The model under review builds one solid part; all positions refer to its coordinate system, in mm. Round coordinates to 2 decimals unless told otherwise and drop trailing zeros. Order: outer loops, then holes, each group sorted by start corner. A loop starts at its lowest first (then second) coordinate and runs counter-clockwise, first axis right, second up. Notation, with made-up numbers: M 28,-33.75 L 52,-33.75 A26 ccw 52,-17.75 Z; hole C -40,-24.5 d4. An arc over 180 degrees is marked long. Answer as a JSON object with one key per item and string values. Group by question number.
1) Insertion check: pin 1 Ø1.5 at (y, z) = (11, 0.5) entering from +X; pin 2 Ø5 at (x, y) = (7.5, 9.5) entering from +Z. Each pin has a flat end and moves straight along its axis. Give the tip position at first contact, or say it passes through.
2) Consider section A-A, the plane z = 2.1. Write out the cut boundary in (x, y).
3) To check wall thickness, follow line 1 (X direction, y = 2.5, z = 1.8); line 2 (Y direction, x = 5, z = 3.75); line 3 (X direction, y = 7, z = 3.1). State the ranges of each line that lie inside material, in increasing order.
4) Consider section C-C, the plane x = 6. Write out the cut boundary in (y, z).
5) Consider section B-B, the plane y = 2. Write out the cut boundary in (x, z), then the cut area to 3 significant figures.
```python
from build123d import *

# Parameters (mm, degrees)
BOSS_EXTRUDE1_DEPTH = 4.7625


with BuildPart() as part:
    # Sketch1 → Boss-Extrude1 (new body)
    with BuildSketch(Plane.XY):
        with BuildLine():
            Line((0, 0), (12.758578644, 0))
            ThreePointArc((12.758578644, 0), (12.850966597, 0.061731657), (12.829289322, 0.170710678))
            Line((12.829289322, 0.170710678), (0.170710678, 12.829289322))
            ThreePointArc((0.170710678, 12.829289322), (0.061731657, 12.850966597), (0, 12.758578644))
            Line((0, 12.758578644), (0, 0))
        make_face()
    extrude(amount=BOSS_EXTRUDE1_DEPTH)


solid = part.part
```
Results list:
{
 "1": {"pin 1": "x = 2.75", "pin 2": "through"},
 "2": {"outline": "M 0,0 L 12.76,0 A0.1 ccw 12.83,0.17 L 0.17,12.83 A0.1 ccw 0,12.76 Z"},
 "3": {"line 1": "0 to 10.5", "line 2": "0 to 8", "line 3": "0 to 6"},
 "4": {"outline": "M 0,0 L 7,0 L 7,4.76 L 0,4.76 Z"},
 "5": {"outline": "M 0,0 L 11,0 L 11,4.76 L 0,4.76 Z", "area": "52.4 mm^2"}
}
